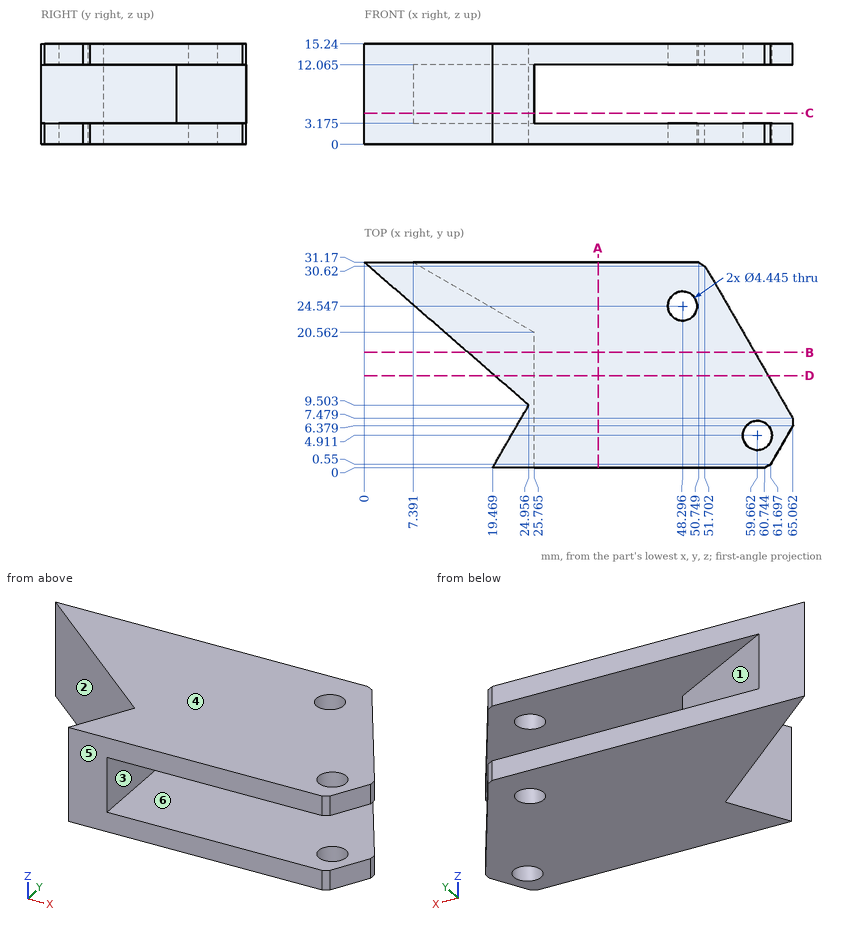
Source: three-view drawing plus pictorial views. Frame: mm from the lowest corner of the part. A direction names the side the tool comes from. Coordinates: 2 decimals unless noted, no trailing zeros. Loops run counter-clockwise (first coordinate to the right, second up) from the corner with the lowest first, then second, coordinate; pieces in that order, holes last. Notation, with made-up numbers: (7, 64.25) -> (27, 64.25) arc R19 ccw to (27, 71.25) -> close; hole circle Ø1 at (37.5, -12). An arc over 180 degrees is marked (long way). Answer in a Markdown table with one row per item. Add a question column.
Q1. Section A-A on x = 35.5. Return the cut outline in (y, z) (1 decimal).
Q2. Section D-D on y = 14. Return the cut outline in (x, z) (1 decimal), and give its area (3 significant figures).
Q3. Section B-B on y = 17.5. Return the cut outline in (x, z) (1 decimal).
Q4. Pull-direction query (Z, two-part tool) for the marked faces 4, 5 and 6; classes: pulls with the +Z half, pulls with the -Z half, needs draft (parallel to the pull), parting line crosses it, or undercut.
Q5. Contact query for flat-ended pins moving along their axis: pin 1 Ø2 at (y, z) = (27, 4.5) entering from -X; pin 2 Ø3 at (y, z) = (13.5, 5.5) entering from -X (1 decimal); pin 3 Ø2.5 at (y, z) = (5.5, 8.5) entering from +X (1 decimal). Output: stop coordinate, or through.
Q6. Ray query, line 1 along Z through (x, y) = (34.5, 15.5) (1 decimal); line 2 along X through (y, z) = (16, 5.75) (1 decimal); line 3 along X through (y, z) = (2.5, 2.75). Return the intervals inside material, ascending.
Q7. Reachability of the marked faces 1, 2 and 3 from +Z, -Z, +X, -X, +Y, -Y: full face, straight path, thin tool, end or side. Return the list, or none.
Q8. Section C-C on z = 4.75. Return the cut outline in (x, y) (1 decimal), and give its area (3 significant figures).
Computed values:
| question | item | result |
|---|---|---|
| 1 | outline | (0, 0) -> (31.2, 0) -> (31.2, 3.2) -> (0, 3.2) -> close; (0, 12.1) -> (31.2, 12.1) -> (31.2, 15.2) -> (0, 15.2) -> close |
| 2 | outline | (19.8, 0) -> (61.3, 0) -> (61.3, 3.2) -> (25.8, 3.2) -> (25.8, 12.1) -> (61.3, 12.1) -> (61.3, 15.2) -> (19.8, 15.2) -> close |
| 2 | area | 317 mm^2 |
| 3 | outline | (15.7, 0) -> (59.3, 0) -> (59.3, 3.2) -> (25.8, 3.2) -> (25.8, 12.1) -> (59.3, 12.1) -> (59.3, 15.2) -> (15.7, 15.2) -> close |
| 4 | face 4 | pulls with the +Z half |
| 4 | face 5 | needs draft |
| 4 | face 6 | undercut |
| 5 | pin 1 | stops at x = 3.65 |
| 5 | pin 2 | stops at x = 18.6 |
| 5 | pin 3 | stops at x = 25.8 |
| 6 | line 1 | z = 0 to 3.2, 12.1 to 15.2 |
| 6 | line 2 | x = 17.5 to 25.8 |
| 6 | line 3 | x = 20.91 to 62.82 |
| 7 | face 1 | +X, +Y |
| 7 | face 2 | +Z, -Z, -X |
| 7 | face 3 | +X, +Y, -Y |
| 8 | outline | (0, 31.2) -> (25, 9.5) -> (19.5, 0) -> (25.8, 0) -> (25.8, 20.6) -> (7.4, 31.2) -> close |
| 8 | area | 224 mm^2 |
